Here's how the part is built. I have some questions about the finished solid (model axes, mm). Face numbers are marked on the shaded views. A direction names the side the tool comes from. Coordinates: 2 decimals unless noted, no trailing zeros. Order: outer loops, then holes, each group sorted by start corner. A loop starts at its lowest first (then second) coordinate and runs counter-clockwise, first axis right, second up. Notation, with made-up numbers: M 75,66 L 106,66 A18 ccw 106,97 Z; hole C 86.5,-5.75 d5. An arc over 180 degrees is marked long. One line per question, with ' | ' between items. Start each with the question number.
```python
from build123d import *

# Parameters (mm, degrees)
BOSS_EXTRUDE1_DEPTH      = 10
BOSS_EXTRUDE2_DEPTH      = 15
BOSS_EXTRUDE2_DEPTH_BACK = 5
SKETCH1_3_R              = 3
SKETCH2_R                = 1.5
CUT_EXTRUDE1_DEPTH       = 32.288975694
BOSS_EXTRUDE3_DEPTH      = 5
BOSS_EXTRUDE3_DEPTH_BACK = 15
SKETCH3_R                = 3


with BuildPart() as part:
    # Sketch1 → Boss-Extrude1 (new body)
    with BuildSketch(Plane.XY):
        with BuildLine():
            Line((-15, 7.5), (-15, -7.5))
            Line((-15, -7.5), (-2.846049894, -11.551316702))
            ThreePointArc((-2.846049894, -11.551316702), (0, -9.5), (2.846049894, -11.551316702))
            Line((2.846049894, -11.551316702), (15, -7.5))
            Line((15, -7.5), (15, 7.5))
            Line((15, 7.5), (-15, 7.5))
        make_face()
    extrude(amount=BOSS_EXTRUDE1_DEPTH)

    # Sketch1_3 → Boss-Extrude2 (add, two sides: drawn at the far end of the back side and taken through both)
    with BuildSketch(Plane.XY.offset(-BOSS_EXTRUDE2_DEPTH_BACK)):
        with Locations((0, -12.5)):
            Circle(SKETCH1_3_R)
    extrude(amount=BOSS_EXTRUDE2_DEPTH + BOSS_EXTRUDE2_DEPTH_BACK)

    # Sketch2 → Cut-Extrude1 (cut, through all)
    with BuildSketch(Plane(origin=(0, 7.5, 0), x_dir=(1, 0, 0), z_dir=(0, 1, 0))):
        with Locations(Location((-9, -5, 0), (0, 0, 270))):
            Circle(SKETCH2_R)
        with Locations((9, -5)):
            Circle(SKETCH2_R)
    extrude(amount=-CUT_EXTRUDE1_DEPTH, mode=Mode.SUBTRACT)

    # Sketch3 → Boss-Extrude3 (add, two sides: drawn at the far end of the back side and taken through both)
    with BuildSketch(Plane(origin=(0, 0, 0), x_dir=(-1, 0, 0), z_dir=(0, 0, -1)).offset(-BOSS_EXTRUDE3_DEPTH_BACK)):
        with Locations((0, 7.5)):
            Circle(SKETCH3_R)
    extrude(amount=BOSS_EXTRUDE3_DEPTH + BOSS_EXTRUDE3_DEPTH_BACK)


solid = part.part
```
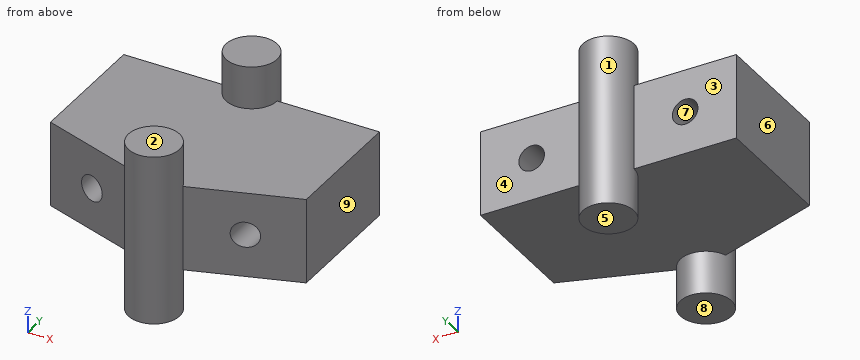
1. Which directions (+Z, -Z, +X, -X, +Y, -Y) give clear straight access to the entire face, cutting with the end or side of a thin tool? Please do the marked faces 1, 2, 3, 4 and 5.
2. Imagine slicing it at B-B (y = -5.5). List the corners of the cut face in (x, z) for me, then the cut area to 3 significant figures.
3. I need wall thicknesses on line 1 (X direction, y = 1.5, z = 5); line 2 (Z direction, x = -9, y = 1.5); line 3 (Z direction, x = -12.5, y = 5.5). Which ranges of each line are inside material? Lowest first, please.
4. Imagine slicing it at D-D (z = -3). List the corners of the cut face in (x, y) for me.
5. Imagine slicing it at C-C (x = 0). List the corners of the cut face in (y, z) for me.
6. Will these pins go through, and if not, where does the flat tip stop? pin 1 (4 mm diameter, centred on x = 2.5, z = 12, fed in from -Y); pin 2 (5.5 mm diameter, centred on x = 0.5, y = -5.5, fed in from -Z); pin 3 (5 mm diameter, centred on x = -7, z = 2.5, fed in from +Y); pin 4 (8 mm diameter, centred on x = -4, z = 0, fed in from +Y).
7. We'd pull the mould along X, two halves only. Please class the marked faces 6, 7, 8 and 9: released by +X, released by -X, zero draft, split by the parting line, or undercut.
8. Imagine slicing it at A-A (z = 5). List the corners of the cut face in (x, y) for me.
Entries:
1) face 1: none | face 2: +Z, +X, -X, +Y, -Y | face 3: +Z, -Z, -X, +Y | face 4: +Z, -Z, +X, +Y | face 5: -Z, +X, -X, +Y, -Y
2) outline: M -15,0 L 15,0 L 15,10 L -15,10 Z; hole C -9,5 d3; hole C 9,5 d3 | area: 286 mm²
3) line 1: -15 to -10.5, -7.5 to 7.5, 10.5 to 15 | line 2: 0 to 3.5, 6.5 to 10 | line 3: 0 to 10
4) outline: C 0,-12.5 d6; C 0,7.5 d6
5) outline: M -15.5,-5 L -9.5,-5 L -9.5,0 L 4.5,0 L 4.5,-5 L 10.5,-5 L 10.5,15 L 4.5,15 L 4.5,10 L -9.5,10 L -9.5,15 L -15.5,15 Z
6) pin 1: y = -15.46 | pin 2: z = 0 | pin 3: y = 7.5 | pin 4: y = 10.5
7) face 6: released by -X | face 7: undercut | face 8: zero draft | face 9: released by +X
8) outline: M -15,-7.5 L -10.5,-9 L -10.5,7.5 L -15,7.5 Z; M -7.5,-10 L -2.85,-11.55 A3 ccw long 2.85,-11.55 L 7.5,-10 L 7.5,7.5 L 3,7.5 A3 ccw -3,7.5 L -7.5,7.5 Z; M 10.5,-9 L 15,-7.5 L 15,7.5 L 10.5,7.5 Z
